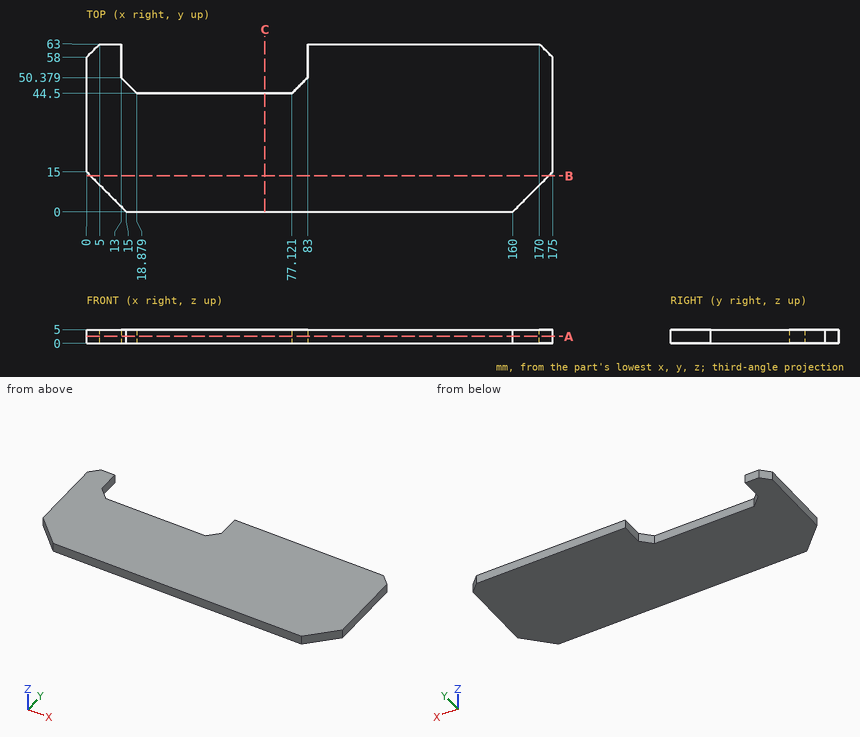
Geometry check sheet. Reference: drawing and pictorial views, mm from the part's lowest x, y, z. Round coordinates to 2 decimals unless told otherwise and drop trailing zeros. Write each loop counter-clockwise with the first axis right and the second up, starting at its lowest first coordinate (ties: lowest second). Pieces come first, ordered by that corner, then holes. Notation, with made-up numbers: (11.25, 25) -> (44.25, 25) arc R22 cw to (44.25, 56) -> close; hole circle Ø5 at (27.25, 24.25). An arc over 180 degrees is marked (long way). Answer as CSV lines item,"result". Start each with the question number.
1) Section check C-C on x = 67. Enter the section's corners in (y, z).
2) Section check B-B on y = 13.5. Enter the section's corners in (x, z), and give its area (3 significant figures).
3) Section check A-A on z = 2.55. Enter the section's corners in (x, y), and give its area (3 significant figures).
4) Go/stop test with flat-tipped pins: P1, Ø1, axis at y = 8, z = 3, coming from the +X side; P2, Ø1.5, axis at x = 34, z = 2, coming from the +Y side. Record where each tip stops, or that it passes through.
5) Material ranges on line 1 (X direction, y = 54, z = 2.65); line 2 (Y direction, x = 37.5, z = 3.6); line 3 (X direction, y = 50, z = 2.65), recorded low to high. Write a range as from..to.
Found:
1,outline,"(0, 0) -> (44.5, 0) -> (44.5, 5) -> (0, 5) -> close"
2,outline,"(1.5, 0) -> (173.5, 0) -> (173.5, 5) -> (1.5, 5) -> close"
2,area,"860 mm^2"
3,outline,"(0, 15) -> (15, 0) -> (160, 0) -> (175, 15) -> (175, 58) -> (170, 63) -> (83, 63) -> (83, 50.38) -> (77.12, 44.5) -> (18.88, 44.5) -> (13, 50.38) -> (13, 63) -> (5, 63) -> (0, 58) -> close"
3,area,"9,510 mm^2"
4,P1,"stops at x = 168.5"
4,P2,"stops at y = 44.5"
5,line 1,"x = 0..13, 83..175"
5,line 2,"y = 0..44.5"
5,line 3,"x = 0..13.38, 82.62..175"
